Autodesk Inventor part; units mm, degrees
ref_plane "YZ Plane" through (0, 0, 0) normal (1, 0, 0) x (0, 1, 0)
ref_plane "XZ Plane" through (0, 0, 0) normal (0, 1, 0) x (-1, 0, 0)
ref_plane "XY Plane" through (0, 0, 0) normal (0, 0, 1) x (1, 0, 0)
sketch "Sketch1" plane through (0, 0, 0) normal (0, 0, 1) x (1, 0, 0)
  circle A0 centre (0, 0) radius 7.15
  line L0 (-7.15, 0) -> (-3.575, 6.1921)
  line L1 (-3.575, 6.1921) -> (3.575, 6.1921)
  line L2 (3.575, 6.1921) -> (7.15, 0)
  line L3 (7.15, 0) -> (3.575, -6.1921)
  line L4 (3.575, -6.1921) -> (-3.575, -6.1921)
  line L5 (-3.575, -6.1921) -> (-7.15, 0)
  dimension "d0" = 14.3
extrude "Extrusion1" add sketch "Sketch1" along normal mid plane 9.3 contours L3 L4 L5 L0 L1 L2
sketch "Sketch2" plane through (0, 0, 4.65) normal (0, 0, 1) x (1, 0, 0)
  point P0 (0, 0)
hole "Hole1" at (0, 0, 4.65) direction (0, 0, -1) diameter 6.75 end through all
thread "Thread1"
fillet "Fillet1" radius 1.5875 6 edges at (-3.575, -6.1921, 0) (-7.15, 0, 0) (-3.575, 6.1921, 0) (3.575, 6.1921, 0) (7.15, 0, 0) (3.575, -6.1921, 0)
properties part number "CNC-1.1v-B-1-( nut )"
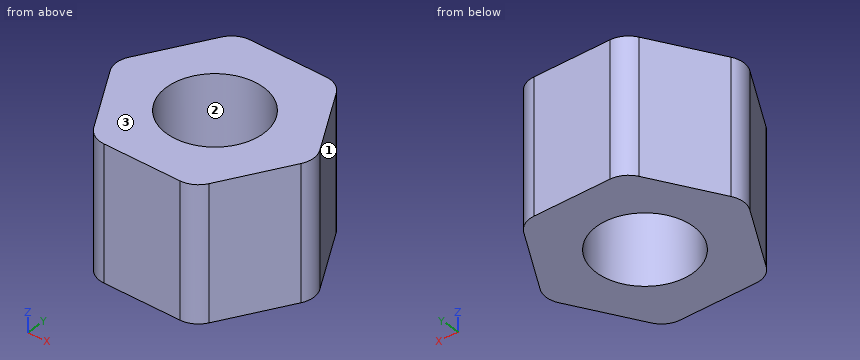
Geometry check sheet. Reference: the model listing, model coordinates, mm. Face numbers are marked on the shaded views. Give positions to 0.01 mm unless a question says otherwise; leave off trailing zeros. Order: outer loops, then holes, each group sorted by start corner. A loop starts at its lowest first (then second) coordinate and runs counter-clockwise, first axis right, second up.
1. Sectioned sample at C-C (y = 0). Record the boundary of the cut face in (x, z) (3 decimals).
Completed:
outline: (-6.904, -4.65) - (-3.375, -4.65) - (-3.375, 4.65) - (-6.904, 4.65) - close; (3.375, -4.65) - (6.904, -4.65) - (6.904, 4.65) - (3.375, 4.65) - close
2. Scan lines: line 1 (X direction, y = 0, z = 1) (3 decimals); line 2 (Y direction, x = 0, z = 1.5) (3 decimals); line 3 (X direction, y = -2.25, z = 2.25). Record each from-to range of solid material in increasing order.
Completed:
line 1: x = -6.904 to -3.375, 3.375 to 6.904
line 2: y = -6.192 to -3.375, 3.375 to 6.192
line 3: x = -5.85 to -2.52, 2.52 to 5.85
3. Sectioned sample at D-D (x = 5.5). Record the boundary of the cut face in (y, z), then the cut area to 3 significant figures.
Completed:
outline: (-2.86, -4.65) - (2.86, -4.65) - (2.86, 4.65) - (-2.86, 4.65) - close
area: 53.2 mm2
4. Draft check along Y on the marked faces 1, 2 and 3. Enter one of: pulls with the +Y half, pulls with the -Y half, needs draft (parallel to the pull), parting line crosses it, or undercut.
Completed:
face 1: pulls with the +Y half
face 2: undercut
face 3: needs draft
5. Sectioned sample at A-A (x = 0). Record the boundary of the cut face in (y, z) (3 decimals), then the cut area to 3 significant figures.
Completed:
outline: (-6.192, -4.65) - (-3.375, -4.65) - (-3.375, 4.65) - (-6.192, 4.65) - close; (3.375, -4.65) - (6.192, -4.65) - (6.192, 4.65) - (3.375, 4.65) - close
area: 52.4 mm2
6. Depth check by flat-ended pin: pin 1 (3 mm diameter, centred on y = 3.5, z = -1, fed in from +X); pin 2 (1 mm diameter, centred on x = -2.5, y = -2, fed in from +Z); pin 3 (5 mm diameter, centred on y = -3, z = 2.5, fed in from -X). Enter the tip coordinate at first touch or a pass-through.
Completed:
pin 1: stops at x = 6
pin 2: stops at z = 4.65
pin 3: stops at x = -6.82
